Read the model definition and answer for the solid it produces. Units are mm, in the model's axes. Coordinates: 2 decimals unless noted, no trailing zeros. Order: outer loops, then holes, each group sorted by start corner. A loop starts at its lowest first (then second) coordinate and runs counter-clockwise, first axis right, second up. Notation, with made-up numbers: (-21.5, 10) - (17.5, 10) arc R29 ccw to (17.5, 42) - close; hole circle Ø11 at (88.25, 10.25). An arc over 180 degrees is marked (long way). Write item = value, one per line.
from build123d import *

# Parameters (mm, degrees)
F0_W     = 155
F0_H     = 100
F1_DEPTH = 18
F2_SIZE  = 20
F4_R     = 5


with BuildPart() as f1:
    # F0 (on Top) → F1 (new body)
    with BuildSketch(Plane.XY):
        with Locations((77.5, 50)):
            Rectangle(F0_W, F0_H)
    extrude(amount=F1_DEPTH)

    # F2
    f2_edges = [f1.edges().sort_by_distance(p)[0] for p in [
        (155, 100, 9),
        (155, 0, 9),
        (0, 100, 9),
        (0, 0, 9),
    ]]
    chamfer(f2_edges, length=F2_SIZE)

    # F6: sweep along a path in F5
    with BuildLine(Plane.XY.offset(18)) as f6_path:
        Line((0, 80), (20, 100))
        Line((20, 100), (135.0186169147, 100))
        Line((135.0186169147, 100), (155, 80))
        Line((155, 80), (155, 20))
        Line((155, 20), (135, 0))
        Line((135, 0), (20, 0))
        Line((20, 0), (0, 20))
        Line((0, 20), (0, 25))
        Line((0, 25), (0, 80))
    # F4 (on offset) → F6 (sweep, cut)
    with BuildSketch(Plane.XZ.offset(-25)):
        with Locations((0, 18)):
            Circle(F4_R)
    sweep(path=f6_path.line, transition=Transition.RIGHT, mode=Mode.SUBTRACT)


solid = f1.part
1) The part is cut by section A-A (x = 60). Determine the outline of the cut face in (y, z), and give its area (3 significant figures).
Returned:
outline = (0, 0) - (100, 0) - (100, 13) arc R5 cw to (95, 18) - (5, 18) arc R5 cw to (0, 13) - close
area = 1,760 mm^2
2) Straight lines are drawn through the part: line 1 along Y through (x, z) = (106.5, 15); line 2 along X through (y, z) = (7, 10.25); line 3 along Y through (x, z) = (20.5, 14.75). For each, find the intervals that lie inside material, in ascending order. Write a range as from..to.
Returned:
line_1 = 4..96
line_2 = 13..142
line_3 = 4.87..95.13
3) A flat-ended cylindrical pin translates along its axis: pin 1 Ø1 at (y, z) = (89.5, 9.5) entering from -X. Find the tip coordinate at first contact, or state that the pin passes through.
Returned:
pin_1 = 9
4) The part is cut by section B-B (z = 9). Determine the outline of the cut face in (x, y).
Returned:
outline = (0, 20) - (20, 0) - (135, 0) - (155, 20) - (155, 80) - (135, 100) - (20, 100) - (0, 80) - close
5) The part is cut by section C-C (z = 16). Determine the outline of the cut face in (x, y).
Returned:
outline = (4.58, 21.9) - (21.9, 4.58) - (133.1, 4.58) - (150.42, 21.9) - (150.42, 78.1) - (133.12, 95.42) - (21.9, 95.42) - (4.58, 78.1) - close
